Can you work these out from the model? Positions are in its coordinate system, mm. A direction names the side the tool comes from. Coordinates: 2 decimals unless noted, no trailing zeros. Order: outer loops, then holes, each group sorted by start corner. A loop starts at its lowest first (then second) coordinate and runs counter-clockwise, first axis right, second up. Notation, with made-up numbers: (-36, 49.5) - (0, 49.5) arc R22 ccw to (0, 57.5) - close; hole circle Ø6 at (24, 29.5). An arc over 180 degrees is marked (long way). Use a Markdown table: item, result. Add a question column.
(1) On a 3-axis mill with a long thin cutter (end or side, diameter ignored), from which of +Z, -Z, +X, -X, +Y, -Y can I reach the whole of each face in a straight line? I mean faces 4 (the cylindrical face through (3.755, 11.923, 91.634)), 5 (the flat face through (-5, 0, -100)), 6 (the cylindrical face through (-3.755, 11.923, -91.634)). Say none if no direction works.
(2) I want a section at A-A (z = 53). List the corners of the cut face in (x, y) for me.
(3) I want a section at B-B (z = 12). List the corners of the cut face in (x, y) for me, and give its area (3 significant figures).
(4) If I drill on L1, parallel to X at y = 0, z = 54; L2, parallel to Y at x = 0, z = 79.5, over which ranges is the centre line in solid material (lowest first)? Write a range as [from, to].
(5) We'd pull the mould along Y, two halves only. Please class faces 1 (the flat face through (-5, 0, 100)), 2 (the cylindrical face through (15.02, 47.69, -1.08)), 3 (the cylindrical face through (2.83, 3.087, -70.087)): pulls with the +Y half, pulls with the -Y half, needs draft (parallel to the pull), parting line crosses it, or undercut.
(6) For pin 1 Ø8 at (x, y) = (-30, 20) entering from -Z; pin 2 Ø1 at (y, z) = (21.5, 41.5) entering from +X; pin 3 Ø1.5 at (x, z) = (-38, 34.5) entering from -Y; pin 4 Ø13.5 at (x, y) = (0, 0) entering from -Z, each with a flat end and sliding along its axis, tell me the tip position at first contact or that it passes through.
Autodesk Inventor part; units mm, degrees
ref_plane "YZ Plane" through (0, 0, 0) normal (1, 0, 0) x (0, 1, 0)
ref_plane "XZ Plane" through (0, 0, 0) normal (0, 1, 0) x (-1, 0, 0)
ref_plane "XY Plane" through (0, 0, 0) normal (0, 0, 1) x (1, 0, 0)
sketch "草圖1" plane through (0, 0, 0) normal (1, 0, 0) x (0, 1, 0)
  line L0 (-26.8, 0) -> (62.8, 0)
  line L1 (0, -120) -> (0, 20)
  line L2 (-14, -100) -> (14, -100)
  line L3 (0, -100) -> (12.5, -100)
  line L4 (12.5, -100) -> (12.5, -83.5)
  line L5 (12.5, -83.5) -> (0, -83.5)
  line L6 (0, -83.5) -> (0, -100)
  line L7 (12.5, -83.5) -> (50, -80.2192)
  line L8 (12.5, -83.5) -> (37.1972, -83.5) construction
  line L9 (50, -80.2192) -> (50, 0)
  line L10 (50, 0) -> (0, 0)
  line L11 (0, 0) -> (0, -83.5)
  dimension "d0" = 100
  dimension "d1" = 12.5
  dimension "d2" = 16.5
  dimension "d3" = 0
  dimension "d4" = 5
  dimension "d5" = 50
revolve "迴轉1" add sketch "草圖1" angle 360 about axis through (0, 0, 0) along (0, 0, -1)
mirror "鏡射1" about plane through (0, 50, 0) normal (0, 0, 1) of "迴轉1"
chamfer "倒角1" distance 3 angle 45 2 edges at (0, -50, 80.2192) (0, -50, -80.2192)
hole "孔1" at (0, 0, 100) direction (0, 0, -1) diameter 8.376 depth 59 tip angle 118
ref_plane "工作平面1" through (0, 0, 0) normal (0, 0, 1) x (1, 0, 0)
ref_plane "工作平面2" through (0, 0, 0) normal (0, 0, -1) x (-1, 0, 0)
mirror "鏡射2" about plane through (0, 0, 0) normal (0, 0, 1) of "孔1"
properties part number "exercise3-11"
Answers follow:
| question | item | result |
|---|---|---|
| 1 | face 4 | +Z |
| 1 | face 5 | -Z, +X, -X, +Y, -Y |
| 1 | face 6 | -Z |
| 2 | outline | circle Ø100 at (0, 0); hole circle Ø8.38 at (0, 0) |
| 3 | outline | circle Ø100 at (0, 0) |
| 3 | area | 7,850 mm² |
| 4 | L1 | x = [-50, -4.19], [4.19, 50] |
| 4 | L2 | y = [-47.91, -4.19], [4.19, 47.91] |
| 5 | face 1 | needs draft |
| 5 | face 2 | parting line crosses it |
| 5 | face 3 | undercut |
| 6 | pin 1 | stops at z = -81.79 |
| 6 | pin 2 | stops at x = 45.38 |
| 6 | pin 3 | stops at y = -33.35 |
| 6 | pin 4 | stops at z = -100 |
